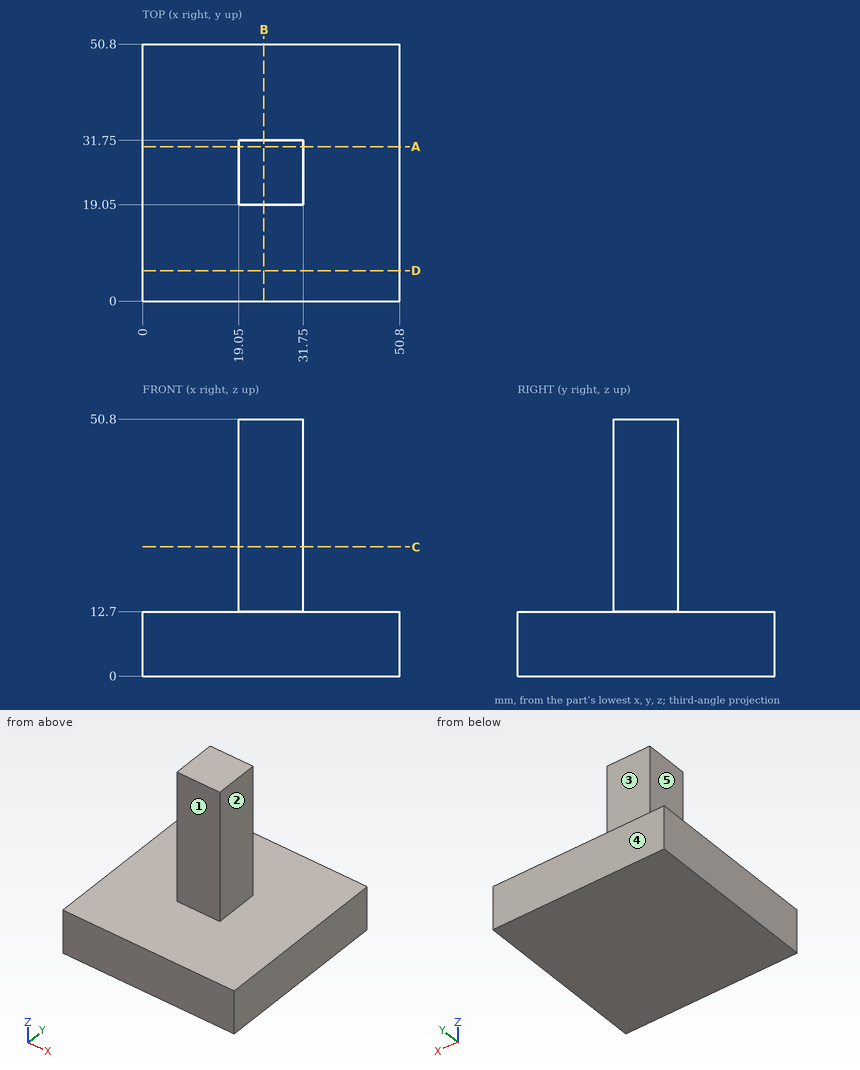
Design review of the part shown in the three views and the two pictorial views. Dimensions are in mm from the part's minimum x, y and z. A direction names the side the tool comes from. Coordinates: 2 decimals unless noted, no trailing zeros. Order: outer loops, then holes, each group sorted by start corner. A loop starts at its lowest first (then second) coordinate and runs counter-clockwise, first axis right, second up.
Item 1: Take a section at C-C, the plane z = 25.5. Write out the cut boundary in (x, y), then the cut area to 3 significant figures.
Item 2: For line 1 (Y direction, x = 22.5, z = 34); line 2 (Z direction, x = 6, y = 3), list the stretches that pass through material, from the lowest coordinate up.
Item 3: Take a section at A-A, the plane y = 30.5. Write out the cut boundary in (x, z).
Item 4: Take a section at D-D, the plane y = 6. Write out the cut boundary in (x, z), then the cut area to 3 significant figures.
Item 5: For the marked faces 1, 2, 3, 4 and 5, list the 3-axis set-ups (+Z, -Z, +X, -X, +Y, -Y) from which the entire face can be reached by the end or side of a thin tool; tool diameter is ignored.
Item 6: For pin 1 Ø1.5 at (x, y) = (7, 45.5) entering from +Z; pin 2 Ø4 at (x, z) = (27, 24.5) entering from -Y; pin 3 Ø14 at (y, z) = (22.5, 25.5) entering from -X; pin 4 Ø15 at (x, y) = (33.5, 22) entering from +Z, all flat-tipped, find the tip position at first contact; note any pin that passes through.
The answers:
1. outline: (19.05, 19.05) - (31.75, 19.05) - (31.75, 31.75) - (19.05, 31.75) - close
1. area: 161 mm2
2. line 1: y = 19.05 to 31.75
2. line 2: z = 0 to 12.7
3. outline: (0, 0) - (50.8, 0) - (50.8, 12.7) - (31.75, 12.7) - (31.75, 50.8) - (19.05, 50.8) - (19.05, 12.7) - (0, 12.7) - close
4. outline: (0, 0) - (50.8, 0) - (50.8, 12.7) - (0, 12.7) - close
4. area: 645 mm2
5. face 1: +Z, +X, -X, -Y
5. face 2: +Z, +X, +Y, -Y
5. face 3: +Z, +X, -X, +Y
5. face 4: +Z, -Z, +X, -X, +Y
5. face 5: +Z, -X, +Y, -Y
6. pin 1: stops at z = 12.7
6. pin 2: stops at y = 19.05
6. pin 3: stops at x = 19.05
6. pin 4: stops at z = 50.8
